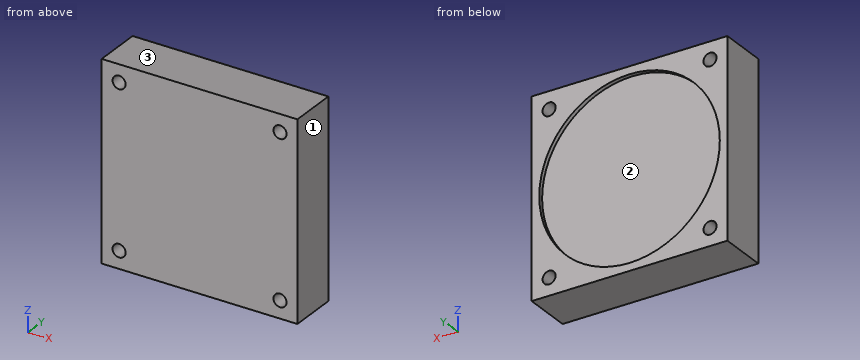
```python
from build123d import *

# Parameters (mm, degrees)
SKETCH1_W           = 45
SKETCH1_H           = 45
SKETCH1_R           = 1.5
BOSS_EXTRUDE1_DEPTH = 11
SKETCH2_R           = 20.75
CUT_EXTRUDE1_DEPTH  = 1


with BuildPart() as part:
    # Sketch1 → Boss-Extrude1 (new body)
    with BuildSketch(Plane(origin=(0, 0, 0), x_dir=(1, 0, 0), z_dir=(0, 1, 0))):
        with Locations((-3.662790698, 9.811046512)):
            Rectangle(SKETCH1_W, SKETCH1_H)
        with Locations(Location((-22.162790698, 28.311046512, 0), (0, 0, 270))):
            Circle(SKETCH1_R, mode=Mode.SUBTRACT)
        with Locations(Location((14.837209302, 28.311046512, 0), (0, 0, 270))):
            Circle(SKETCH1_R, mode=Mode.SUBTRACT)
        with Locations(Location((-22.162790698, -8.688953488, 0), (0, 0, 270))):
            Circle(SKETCH1_R, mode=Mode.SUBTRACT)
        with Locations(Location((14.837209302, -8.688953488, 0), (0, 0, 270))):
            Circle(SKETCH1_R, mode=Mode.SUBTRACT)
    extrude(amount=BOSS_EXTRUDE1_DEPTH)

    # Sketch2 → Cut-Extrude1 (cut)
    with BuildSketch(Plane(origin=(0, 11, 0), x_dir=(1, 0, 0), z_dir=(0, 1, 0))):
        with Locations(Location((-3.662790698, 9.811046512, 0), (0, 0, 270))):
            Circle(SKETCH2_R)
    extrude(amount=-CUT_EXTRUDE1_DEPTH, mode=Mode.SUBTRACT)


solid = part.part
```
Can you work these out from the model? Positions are in its coordinate system, mm. Face numbers are marked on the shaded views. Round coordinates to 2 decimals unless told otherwise and drop trailing zeros. Loops run counter-clockwise (first coordinate to the right, second up) from the corner with the lowest first, then second, coordinate; pieces in that order, holes last. Notation, with made-up numbers: (0.25, 19) -> (57.25, 19) arc R18 ccw to (57.25, 37) -> close; hole circle Ø2 at (55.25, -32.5). An arc over 180 degrees is marked (long way). One line per item, written item: value. Start each with the question number.
1. If we section it at A-A, the plane x = -7: Write out the boundary of the cut face in (y, z).
2. If we mould it in two halves opening along X, with no side actions, what happens to the marked faces 1, 2 and 3? For each: pulls with the +X half, pulls with the -X half, needs draft (parallel to the pull), parting line crosses it, or undercut.
3. If I drill on probe 1 along X at (y, z) = (6, -28.5); probe 2 along X at (y, z) = (3, 8); probe 3 along Y at (x, z) = (13, -7), over which ranges is the centre line in solid material (lowest first)?
4. For pin 1 (3.5 mm diameter, centred on x = 14.84, z = -28.31, fed in from -Y); pin 2 (12.5 mm diameter, centred on x = -10.5, z = -9.5, fed in from +Y), each with a flat end and sliding along its axis, tell me the tip position at first contact or that it passes through.
5. If we section it at B-B, the plane z = -28: Write out the boundary of the cut face in (x, y), then the cut area to 3 significant figures.
6. If we section it at C-C, the plane z = 1: Write out the boundary of the cut face in (x, y).
Calculated:
1. outline: (0, -32.31) -> (11, -32.31) -> (11, -30.29) -> (10, -30.29) -> (10, 10.67) -> (11, 10.67) -> (11, 12.69) -> (0, 12.69) -> close
2. face 1: pulls with the +X half
2. face 2: undercut
2. face 3: needs draft
3. probe 1: x = -26.16 to -23.65, -20.67 to 13.35, 16.33 to 18.84
3. probe 2: x = -26.16 to -23.5, -20.83 to 13.5, 16.17 to 18.84
3. probe 3: y = 0 to 10
4. pin 1: stops at y = 0
4. pin 2: stops at y = 10
5. outline: (-26.16, 0) -> (-23.63, 0) -> (-23.63, 11) -> (-26.16, 11) -> close; (-20.7, 0) -> (13.37, 0) -> (13.37, 11) -> (6.32, 11) -> (6.32, 10) -> (-13.65, 10) -> (-13.65, 11) -> (-20.7, 11) -> close; (16.3, 0) -> (18.84, 0) -> (18.84, 11) -> (16.3, 11) -> close
5. area: 410 mm²
6. outline: (-26.16, 0) -> (18.84, 0) -> (18.84, 11) -> (14.05, 11) -> (14.05, 10) -> (-21.37, 10) -> (-21.37, 11) -> (-26.16, 11) -> close
